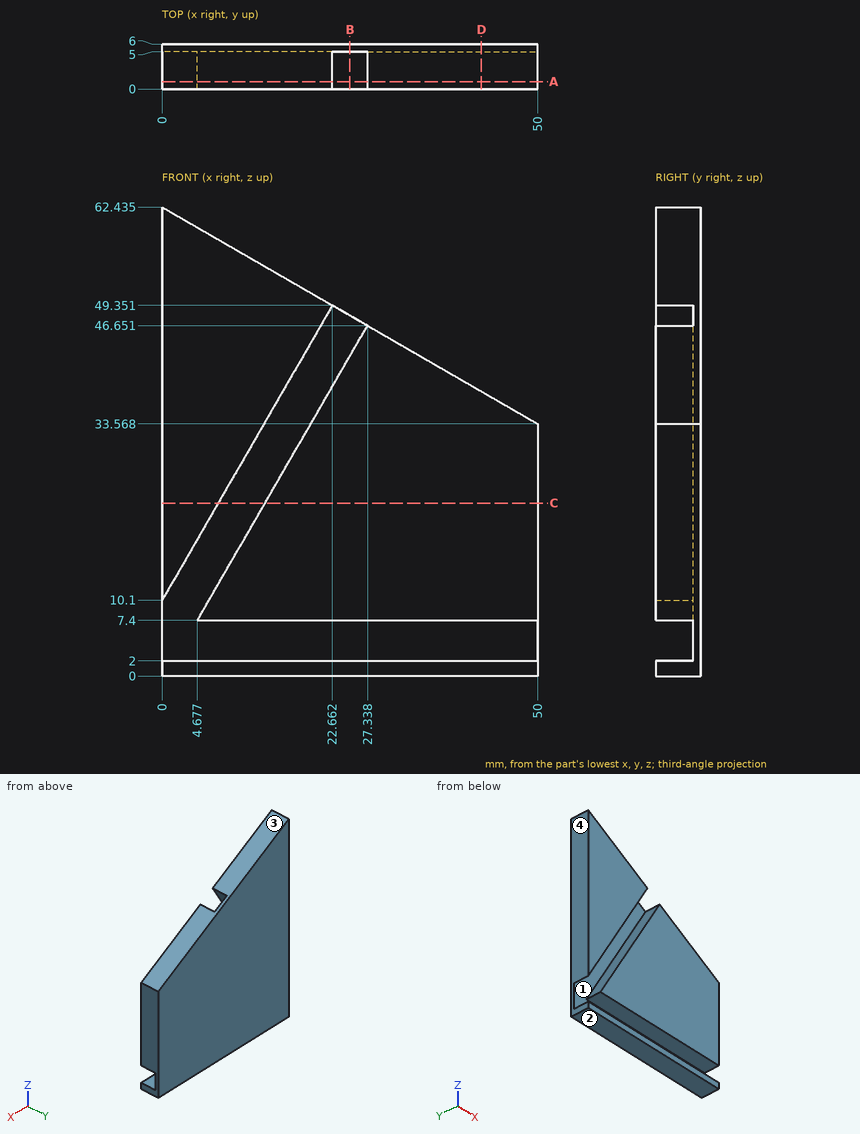
Input: dimensioned drawing with shaded views. Units: mm. Origin: part minimum x, y, z. Coordinates: 2 decimals unless noted, no trailing zeros. Loops run counter-clockwise (first coordinate to the right, second up) from the corner with the lowest first, then second, coordinate; pieces in that order, holes last. Notation, with made-up numbers: M 79.5,44 L 124.5,44 A30 ccw 124.5,70 Z; hole C -37,-13.5 d10. An arc over 180 degrees is marked long. Use a Markdown table: item, result. Add a question column.
1) Section B-B, the plane x = 25. Return the cut outline in (y, z), plus the area to 3 significant figures.
2) Line query: L1, parallel to Z at x = 17, y = 2.3 (1 decimal); L2, parallel to Z at x = 30, y = 4.15 (1 decimal); L3, parallel to Z at x = 13.5, y = 3.7 (1 decimal). Output: solid intervals per line, ascending. Write a range as from..to.
3) Section A-A, the plane y = 1. Return the cut outline in (x, z) (1 decimal), plus the area to 3 significant figures.
4) Section C-C, the plane z = 23. Return the cut outline in (x, y).
5) Draft query along Z for the marked faces 1, 2, 3 and 4. Return one class per face: +Z half, -Z half, draft (parallel to the pull), parting line (faces both ways), or undercut.
6) Section D-D, the plane x = 42.5. Return the cut outline in (y, z).
7) Pin query (flat end, axial travel): P1, Ø2.5, axis at x = 34.5, y = 2, coming from the +Z side. Return the tip coordinate at first contact, or that it passes through.
Answer below:
| question | item | result |
|---|---|---|
| 1 | outline | M 0,0 L 6,0 L 6,48 L 5,48 L 5,42.6 L 0,42.6 L 0,7.4 L 5,7.4 L 5,2 L 0,2 Z |
| 1 | area | 234 mm2 |
| 2 | L1 | 0..2, 7.4..28.7, 39.5..52.6 |
| 2 | L2 | 0..2, 7.4..45.1 |
| 2 | L3 | 0..2, 7.4..22.7, 33.5..54.6 |
| 3 | outline | M 0,0 L 50,0 L 50,2 L 0,2 Z; M 0,10.1 L 22.7,49.4 L 0,62.4 Z; M 4.7,7.4 L 50,7.4 L 50,33.6 L 27.3,46.7 Z |
| 3 | area | 1,880 mm2 |
| 4 | outline | M 0,0 L 7.45,0 L 7.45,5 L 13.68,5 L 13.68,0 L 50,0 L 50,6 L 0,6 Z |
| 5 | face 1 | undercut |
| 5 | face 2 | -Z half |
| 5 | face 3 | +Z half |
| 5 | face 4 | draft |
| 6 | outline | M 0,0 L 6,0 L 6,37.9 L 0,37.9 L 0,7.4 L 5,7.4 L 5,2 L 0,2 Z |
| 7 | P1 | z = 43.24 |
